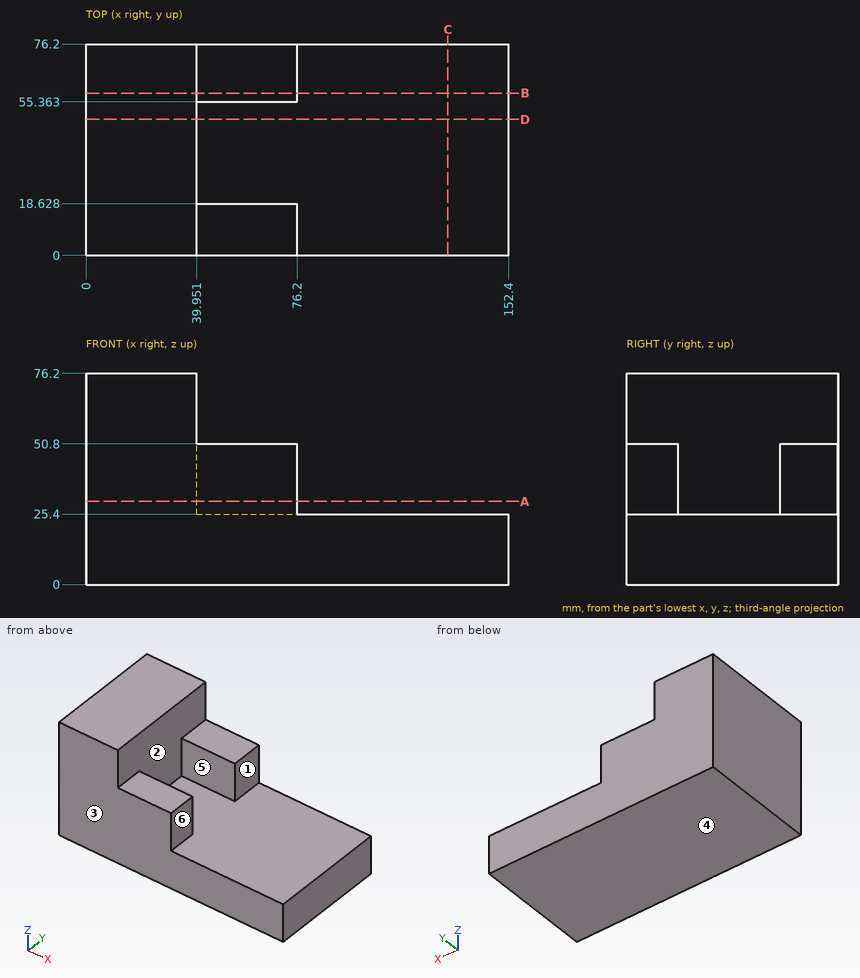
Geometry: see drawing. Coordinates: mm, zero at the bounding-box minimum. A direction names the side the tool comes from. Coordinates: 2 decimals unless noted, no trailing zeros. Order: outer loops, then holes, each group sorted by start corner. A loop starts at its lowest first (then second) coordinate and runs counter-clockwise, first axis right, second up. Notation, with made-up numbers: M 74,24 L 87,24 A13 ccw 87,46 Z; hole C 43,-20 d11. An arc over 180 degrees is marked long. Write item = value, one per line. Start each with the question number.
(1) Line query: line 1 along X through (y, z) = (57, 38.5); line 2 along X through (y, z) = (27, 68); line 3 along Z through (x, y) = (113, 27). Output: solid intervals per line, ascending. Write a range as [from, to].
(2) Section A-A on z = 30. Output: boundary loops of the cut face in (x, y).
(3) Pull-direction query (Y, two-part tool) for the marked faces 1, 2 and 3; classes: released by +Y, released by -Y, zero draft, split by the parting line, or undercut.
(4) Section C-C on x = 130.5. Output: boundary loops of the cut face in (y, z).
(5) Section D-D on y = 49. Output: boundary loops of the cut face in (x, z), and give its area (3 significant figures).
(6) Section B-B on y = 58.5. Output: boundary loops of the cut face in (x, z).
(7) First-contact query: P1, Ø15, axis at y = 54, z = 49, coming from the +X side; P2, Ø6.5, axis at x = 54.5, y = 62.5, coming from the +Z side; P3, Ø1, axis at x = 122.5, y = 56.5, coming from the +Z side; P4, Ø8, axis at x = 126.5, y = 13.5, coming from the -Z side. Flat tips, straight axial feed; report the tip coordinate or a pass-through.
(8) Reachability of the marked faces 4, 5 and 6 from +Z, -Z, +X, -X, +Y, -Y: full face, straight path, thin tool, end or side. Return the list, or none.
Result set:
q1.line_1 = [0, 76.2]
q1.line_2 = [0, 39.95]
q1.line_3 = [0, 25.4]
q2.outline = M 0,0 L 76.2,0 L 76.2,18.63 L 39.95,18.63 L 39.95,55.36 L 76.2,55.36 L 76.2,76.2 L 0,76.2 Z
q3.face_1 = zero draft
q3.face_2 = undercut
q3.face_3 = released by -Y
q4.outline = M 0,0 L 76.2,0 L 76.2,25.4 L 0,25.4 Z
q5.outline = M 0,0 L 152.4,0 L 152.4,25.4 L 39.95,25.4 L 39.95,76.2 L 0,76.2 Z
q5.area = 5,900 mm²
q6.outline = M 0,0 L 152.4,0 L 152.4,25.4 L 76.2,25.4 L 76.2,50.8 L 39.95,50.8 L 39.95,76.2 L 0,76.2 Z
q7.P1 = 76.2
q7.P2 = 50.8
q7.P3 = 25.4
q7.P4 = 0
q8.face_4 = -Z, +X, -X, +Y, -Y
q8.face_5 = +Z, +X
q8.face_6 = +Z, +X, +Y, -Y
